The figure shows three views and two pictorial views of one solid part (mm, origin at its lowest corner). Answer the questions. Coordinates: 2 decimals unless noted, no trailing zeros. Order: outer loops, then holes, each group sorted by start corner. A loop starts at its lowest first (then second) coordinate and runs counter-clockwise, first axis right, second up. Notation, with made-up numbers: (66.5, 21) - (89.5, 21) arc R20 ccw to (89.5, 25) - close; hole circle Ø2 at (8.5, 21). An arc over 180 degrees is marked (long way). Use one line per item in the form item = value.
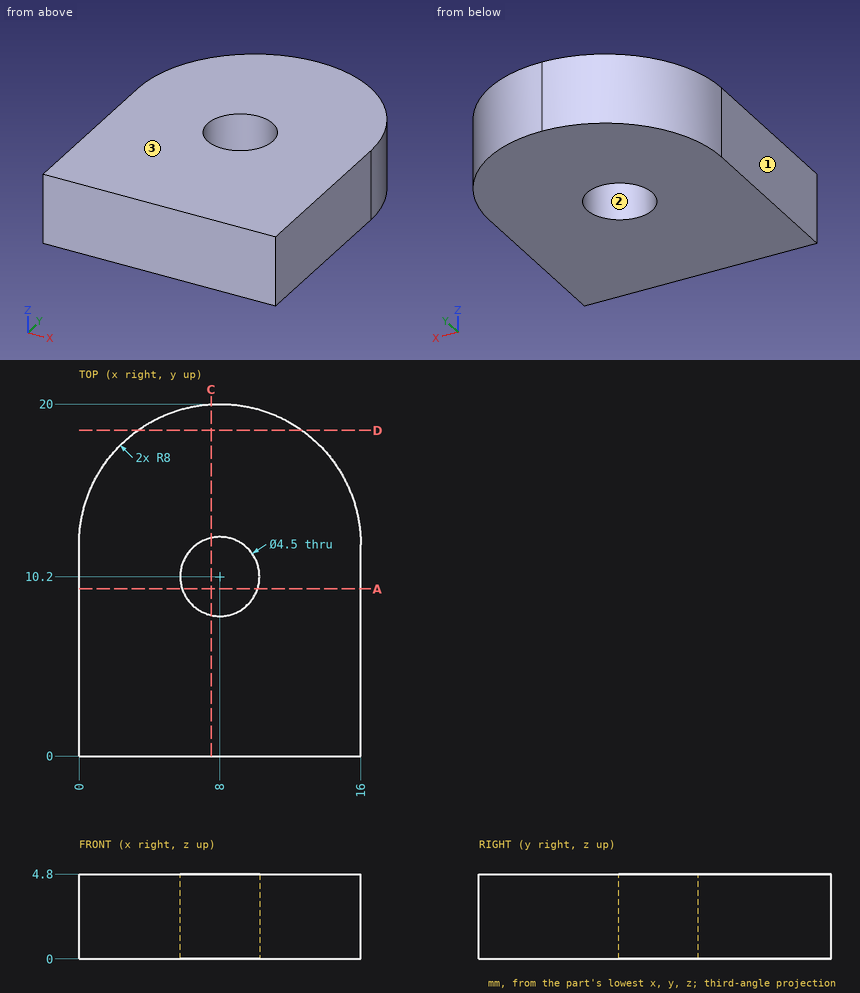
(1) Section A-A, the plane y = 9.5 is taken. Write down the section's boundary in (x, z).
Answer list:
outline = (0, 0) - (5.86, 0) - (5.86, 4.8) - (0, 4.8) - close; (10.14, 0) - (16, 0) - (16, 4.8) - (10.14, 4.8) - close
(2) The mould has two halves that part along X. Classify the marked faces 1, 2 and 3: +X half, -X half, draft (parallel to the pull), parting line (faces both ways), or undercut.
Answer list:
face_1 = -X half
face_2 = undercut
face_3 = draft
(3) Straight lines are drawn through the part: L1, parallel to Y at x = 8, z = 2; L2, parallel to Y at x = 6.5, z = 1.5; L3, parallel to Y at x = 1.75, z = 2.6. For each, find the intervals that lie inside material, in ascending order.
Answer list:
L1 = 0 to 7.95, 12.45 to 20
L2 = 0 to 8.52, 11.88 to 19.86
L3 = 0 to 16.99
(4) Section D-D, the plane y = 18.5 is taken. Write down the section's boundary in (x, z).
Answer list:
outline = (3.34, 0) - (12.66, 0) - (12.66, 4.8) - (3.34, 4.8) - close
(5) Section C-C, the plane x = 7.5 is taken. Write down the section's boundary in (y, z).
Answer list:
outline = (0, 0) - (8.01, 0) - (8.01, 4.8) - (0, 4.8) - close; (12.39, 0) - (19.98, 0) - (19.98, 4.8) - (12.39, 4.8) - close
